Can you work these out from the model? Positions are in its coordinate system, mm. A direction names the side the tool comes from. Round coordinates to 2 decimals unless told otherwise and drop trailing zeros. Loops run counter-clockwise (first coordinate to the right, second up) from the corner with the lowest first, then second, coordinate; pieces in that order, holes last.
(1) Will these pins go through, and if not, where does the flat tip stop? pin 1 Ø6 at (x, y) = (4.5, 100.5) entering from +Z; pin 2 Ø3 at (x, y) = (-48.5, 246) entering from -Z; pin 3 Ø1 at (x, z) = (-68, 99) entering from +Y.
(2) Which directions (+Z, -Z, +X, -X, +Y, -Y) give clear straight access to the entire face, cutting with the end or side of a thin tool? Please do faces 1 (the face through (2, 0, 445)), 2 (the face through (-1, 152.5, -531)).
(3) I want a section at D-D on y = 239. Write out the boundary of the cut face in (x, z).
(4) I want a section at A-A on y = 93.5. Write out the boundary of the cut face in (x, z).
(5) If I drill on line 1 along Z through (x, y) = (-46.5, 344.5); line 2 along Z through (x, y) = (-72, 65.5); line 3 along Y through (x, z) = (60, -531), over which ranges is the centre line in solid material (lowest first)?
(6) I want a section at B-B on x = 0. Write out the boundary of the cut face in (y, z).
(7) I want a section at C-C on z = 0. Write out the boundary of the cut face in (x, y).
from build123d import *

# Parameters (mm, degrees)
BOSS_EXTRUDE1_DEPTH = 120.65
SKETCH2_R           = 97.5
BOSS_EXTRUDE2_DEPTH = 152.5


with BuildPart() as part:
    # Sketch1 → Boss-Extrude1 (new, symmetric)
    with BuildSketch(Plane(origin=(0, 0, 0), x_dir=(0, 0, -1), z_dir=(1, 0, 0))):
        with BuildLine():
            ThreePointArc((508, 0), (0, 508), (-508, 0))
            Line((-508, 0), (-381, 0))
            ThreePointArc((-381, 0), (0, 381), (381, 0))
            Line((381, 0), (508, 0))
        make_face()
    extrude(amount=BOSS_EXTRUDE1_DEPTH, both=True)

    # Sketch2 → Boss-Extrude2 (add)
    with BuildSketch(Plane.XZ):
        with Locations((0, -508)):
            Circle(SKETCH2_R)
    extrude(amount=-BOSS_EXTRUDE2_DEPTH)


solid = part.part
Filled sheet:
1. pin 1: stops at z = 498.56
1. pin 2: stops at z = -445.29
1. pin 3: stops at y = 498.36
2. face 1: +Z, -Z, +X, -X, -Y
2. face 2: -Z, +X, -X, +Y
3. outline: (-120.65, -448.27) - (120.65, -448.27) - (120.65, -296.72) - (-120.65, -296.72) - close; (-120.65, 296.72) - (120.65, 296.72) - (120.65, 448.27) - (-120.65, 448.27) - close
4. outline: (-120.65, -499.32) - (-97.11, -499.32) arc R97.5 ccw (long way) to (97.11, -499.32) - (120.65, -499.32) - (120.65, -369.35) - (-120.65, -369.35) - close; (-120.65, 369.35) - (120.65, 369.35) - (120.65, 499.32) - (-120.65, 499.32) - close
5. line 1: z = -373.34 to -162.73, 162.73 to 373.34
5. line 2: z = -573.74 to -375.33, 375.33 to 503.76
5. line 3: y = 0 to 152.5
6. outline: (0, -605.5) - (152.5, -605.5) - (152.5, -484.57) arc R508 ccw to (0, 508) - (0, 381) arc R381 cw to (0, -381) - close
7. outline: (-120.65, 381) - (120.65, 381) - (120.65, 508) - (-120.65, 508) - close
